Here's the drawing with two shaded views (mm, measured from the low corner). I have some questions. A direction names the side the tool comes from. Coordinates: 2 decimals unless noted, no trailing zeros. Write each loop counter-clockwise with the first axis right and the second up, starting at its lowest first coordinate (ties: lowest second). Pieces come first, ordered by that corner, then holes.
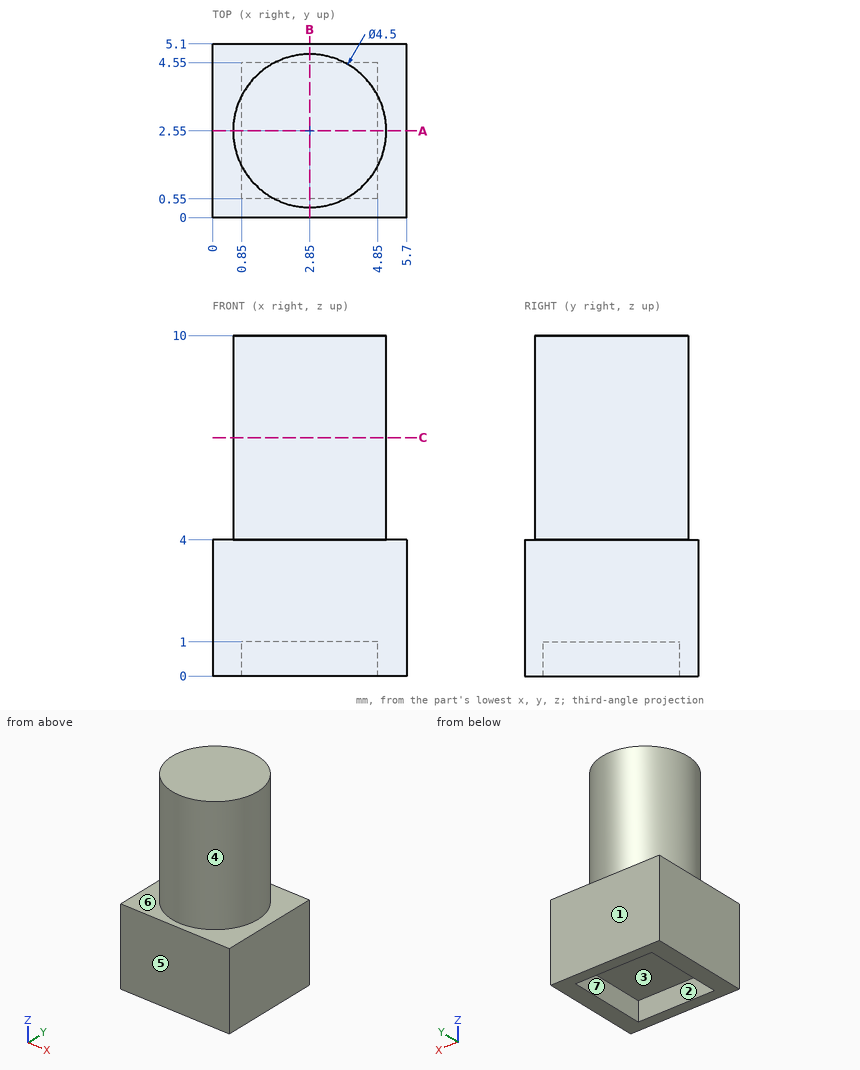
1. I want a section at A-A on y = 2.55. Please give me the cut outline in (x, z).
Verdict:
outline: (0, 0) - (0.85, 0) - (0.85, 1) - (4.85, 1) - (4.85, 0) - (5.7, 0) - (5.7, 4) - (5.1, 4) - (5.1, 10) - (0.6, 10) - (0.6, 4) - (0, 4) - close
2. On a 3-axis mill with a long thin cutter (end or side, diameter ignored), from which of +Z, -Z, +X, -X, +Y, -Y can I reach the whole of each face in a straight line? I mean the marked faces 5, 6 and 7. Say none if no direction works.
Verdict:
face 5: +Z, -Z, +X, -X, -Y
face 6: +Z
face 7: -Z
3. Please list where these lines run through material, in increasing order: line 1 along Z through (x, y) = (3.8, 2.8); line 2 along Z through (x, y) = (5.55, 3.05); line 3 along X through (y, z) = (2.6, 5).
Verdict:
line 1: z = 1 to 10
line 2: z = 0 to 4
line 3: x = 0.6 to 5.1
4. If we mould it in two halves opening along Y, with no side actions, what happens to the marked faces 1, 2, 3 and 4? For each: pulls with the +Y half, pulls with the -Y half, needs draft (parallel to the pull), parting line crosses it, or undercut.
Verdict:
face 1: pulls with the +Y half
face 2: undercut
face 3: undercut
face 4: parting line crosses it
5. I want a section at C-C on z = 7. Please give me the cut outline in (x, y), plus the area to 3 significant figures.
Verdict:
outline: circle Ø4.5 at (2.85, 2.55)
area: 15.9 mm2
6. For pin 1 (1 mm diameter, centred on x = 3, y = 4, fed in from -Z); pin 2 (2 mm diameter, centred on x = 4, y = 1.5, fed in from -Z), each with a flat end and sliding along its axis, tell me the tip position at first contact or that it passes through.
Verdict:
pin 1: stops at z = 1
pin 2: stops at z = 0
7. I want a section at B-B on x = 2.85. Please give me the cut outline in (y, z), plus the area to 3 significant figures.
Verdict:
outline: (0, 0) - (0.55, 0) - (0.55, 1) - (4.55, 1) - (4.55, 0) - (5.1, 0) - (5.1, 4) - (4.8, 4) - (4.8, 10) - (0.3, 10) - (0.3, 4) - (0, 4) - close
area: 43.4 mm2
